Read the model definition and answer for the solid it produces. Units are mm, in the model's axes. A direction names the side the tool comes from. Give positions to 0.01 mm unless a question says otherwise; leave off trailing zeros. Order: outer loops, then holes, each group sorted by start corner. A loop starts at its lowest first (then second) coordinate and runs counter-clockwise, first axis right, second up. Notation, with made-up numbers: M 74,28.25 L 104,28.25 A17 ccw 104,34.25 Z; hole C 49,3 d8. An arc over 180 degrees is marked long. One line per item, written item: value. Start each with the question number.
from build123d import *

# Parameters (mm, degrees)
F1_DEPTH = 127
F2_T     = 6.35
F3_W     = 160.02
F3_H     = 228.6
F3_W_2   = 153.67
F3_H_2   = 222.25
F4_DEPTH = 127
F5_DEPTH = 9.525
F6_R     = 1.5875
F7_DEPTH = 25.4
F8_W     = 29.6064093709
F8_H     = 23.796312511
F9_DEPTH = 25.4


# Not quite as in the source:
# - a shell that OpenCascade refuses in one call is made with other operations: the cavity is built on its own and cut out


with BuildPart() as f1:
    # F0 (on Top) → F1 (new body)
    with BuildSketch(Plane.XY):
        with BuildLine():
            ThreePointArc((-33.8929891586, 6.35), (-32.0331172192, 1.8598719395), (-27.5429891586, 0))
            Line((-27.5429891586, 0), (132.4770108414, 0))
            ThreePointArc((132.4770108414, 0), (136.9671389019, 1.8598719395), (138.8270108414, 6.35))
            Line((138.8270108414, 6.35), (138.8270108414, 234.95))
            ThreePointArc((138.8270108414, 234.95), (136.9671389019, 239.4401280605), (132.4770108414, 241.3))
            Line((132.4770108414, 241.3), (-27.5429891586, 241.3))
            ThreePointArc((-27.5429891586, 241.3), (-32.0331172192, 239.4401280605), (-33.8929891586, 234.95))
            Line((-33.8929891586, 234.95), (-33.8929891586, 6.35))
        make_face()
    extrude(amount=F1_DEPTH)

    # F2: shell of thickness 6.35, made by hand


with BuildPart() as f2_core1:
    # F2_t2: copy of F1
    add(f1.part)

    # the walls: a layer under each face that stays
    f2_faces = [f2_core1.faces().sort_by_distance(p)[0] for p in [
        (52.4670108414, 0, 63.5),
        (138.8270108414, 120.65, 63.5),
        (52.4670108414, 241.3, 63.5),
        (-33.8929891586, 120.65, 63.5),
        (52.4670108414, 120.65, 0),
    ]]
    thicken(f2_faces, amount=-F2_T, mode=Mode.SUBTRACT)


with BuildPart() as f1_1:
    add(f1.part)

    # what is left inside the walls is the cavity
    f2_cavity = [f2_core1.part.solids().sort_by_distance(p)[0] for p in [
        (52.467011, 82.55, 6.4135),
    ]]
    add(f2_cavity, mode=Mode.SUBTRACT)

    # F3 (on face) → F4 (join)
    with BuildSketch(Plane.XY.offset(127)):
        with Locations((52.4670108414, 120.65)):
            Rectangle(F3_W, F3_H)
        with Locations((52.4670108414, 120.65)):
            Rectangle(F3_W_2, F3_H_2, mode=Mode.SUBTRACT)
    extrude(amount=-F4_DEPTH)

    # F3 (on face) → F5 (cut)
    with BuildSketch(Plane.XY.offset(127)):
        with Locations((52.4670108414, 120.65)):
            Rectangle(F3_W, F3_H)
        with Locations((52.4670108414, 120.65)):
            Rectangle(F3_W_2, F3_H_2, mode=Mode.SUBTRACT)
    extrude(amount=-F5_DEPTH, mode=Mode.SUBTRACT)

    # F6 (on face) → F7 (cut)
    with BuildSketch(Plane(origin=(0, 0, 0), x_dir=(1, 0, 0), z_dir=(0, 0, -1))):
        with Locations((-0.9629237612, -29.5858253049)):
            Circle(F6_R)
    extrude(amount=-F7_DEPTH, mode=Mode.SUBTRACT)

    # F8 (on face) → F9 (cut)
    with BuildSketch(Plane(origin=(0, 0, 0), x_dir=(1, 0, 0), z_dir=(0, 0, -1))):
        with Locations((25.6846360862, -31.3592217863)):
            Rectangle(F8_W, F8_H)
    extrude(amount=-F9_DEPTH, mode=Mode.SUBTRACT)


solid = f1_1.part
Q1. This flat-tipped pin is pushed along its axis until it touches: pin 1 (6 mm diameter, centred on x = 100.5, y = 190.5, fed in from +Z). Where does it stop, or does it pass through?
Q2. A tool of negligible diameter and unlimited length cuts with its end or side. For faces 5 (the flat face through (40.488, 32, 3)), 6 (the flat face through (51, 9.525, 63)), 7 (the flat face through (-31, 121, 127)), from which of +Z, -Z, +X, -X, +Y, -Y can it reach the whole face along a straight path? Write none if from no direction.
Q3. Consider probe 1 along X at (y, z) = (74, 29.5); probe 2 along Y at (x, z) = (-23.5, 27) (3 decimals); probe 3 along Z at (x, y) = (64, 178). Determine where each line is inside the solid, lowest interval first.
Q4. Find section C-C, the plane x = 15. Give the vertices of the cut face in (y, z) (3 decimals).
Q5. Determine the mould class of faces 1 (the flat face through (51, 231.775, 63)), 2 (the flat face through (54, 241.3, 63)), 3 (the flat face through (132.477, 119, 122)), 4 (the flat face through (-33.893, 122, 63)) for opening direction X: released by +X, released by -X, zero draft, split by the parting line, or undercut.
Q6. Find section B-B, the plane y = 38.5. Give the vertices of the cut face in (x, z) (3 decimals), then the cut area to 3 significant figures.
Q7. Find section D-D, the plane y = 173.5. Give the vertices of the cut face in (x, z) (3 decimals), then the cut area to 3 significant figures.
Q8. Find section A-A, the plane z = 103.5. Give the vertices of the cut face in (x, y) (3 decimals).
Evaluation:
1. pin 1: z = 6.35
2. face 5: +Z, -Z
2. face 6: +Z
2. face 7: +Z, +X, -X, +Y, -Y
3. probe 1: -33.89 to -24.37, 129.3 to 138.83
3. probe 2: 0 to 9.525, 231.775 to 241.3
3. probe 3: 0 to 6.35
4. outline: M 0,0 L 19.461,0 L 19.461,6.35 L 9.525,6.35 L 9.525,117.475 L 6.35,117.475 L 6.35,127 L 0,127 Z; M 43.257,0 L 241.3,0 L 241.3,127 L 234.95,127 L 234.95,117.475 L 231.775,117.475 L 231.775,6.35 L 43.257,6.35 Z
5. face 1: undercut
5. face 2: zero draft
5. face 3: undercut
5. face 4: released by -X
6. outline: M -33.893,0 L 10.881,0 L 10.881,6.35 L -24.368,6.35 L -24.368,117.475 L -27.543,117.475 L -27.543,127 L -33.893,127 Z; M 40.488,0 L 138.827,0 L 138.827,127 L 132.477,127 L 132.477,117.475 L 129.302,117.475 L 129.302,6.35 L 40.488,6.35 Z
6. area: 3,150 mm2
7. outline: M -33.893,0 L 138.827,0 L 138.827,127 L 132.477,127 L 132.477,117.475 L 129.302,117.475 L 129.302,6.35 L -24.368,6.35 L -24.368,117.475 L -27.543,117.475 L -27.543,127 L -33.893,127 Z
7. area: 3,330 mm2
8. outline: M -33.893,6.35 A6.35 ccw -27.543,0 L 132.477,0 A6.35 ccw 138.827,6.35 L 138.827,234.95 A6.35 ccw 132.477,241.3 L -27.543,241.3 A6.35 ccw -33.893,234.95 Z; hole M -24.368,9.525 L 129.302,9.525 L 129.302,231.775 L -24.368,231.775 Z
